Autodesk Inventor part; units mm, degrees
ref_plane "YZ Plane" through (0, 0, 0) normal (1, 0, 0) x (0, 1, 0)
ref_plane "XZ Plane" through (0, 0, 0) normal (0, 1, 0) x (-1, 0, 0)
ref_plane "XY Plane" through (0, 0, 0) normal (0, 0, 1) x (1, 0, 0)
sketch "Sketch1" plane through (0, 0, 0) normal (0, 1, 0) x (-1, 0, 0)
  circle A0 centre (0, 0) radius 22.606
  circle A1 centre (0, 0) radius 25.273
  dimension "d0" = 45.212
  dimension "d1" = 50.546
extrude "Extrusion1" add sketch "Sketch1" along normal mid plane 25.4
sketch "Sketch5" plane through (0, 0, 0) normal (1, 0, 0) x (0, 1, 0)
  line L0 (-12.7, -22.606) -> (12.7, -22.606)
  arc A0 (0, -25.527) -> (0, -19.685) centre (0, -22.606) ccw
  line L1 (0, -25.527) -> (0, -19.685)
  line L2 (0, -25.527) -> (0, -19.685) construction
  point P0 (0, 0)
  dimension "d7" = 2.921
revolve "Revolution2" add sketch "Sketch5" angle 360 about axis through (0, 0, -25.527) along (0, 0, 1)
properties part number "ExternalMotorizedOuterRing" material "PET Plastic"
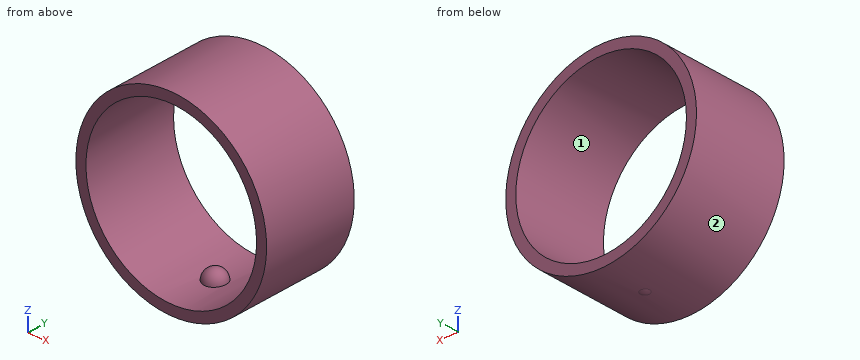
CAD build for the part. Positions are in the model's coordinates, mm. Face numbers are marked on the shaded views. Coordinates: 2 decimals unless noted, no trailing zeros. Order: outer loops, then holes, each group sorted by start corner. A loop starts at its lowest first (then second) coordinate and runs counter-clockwise, first axis right, second up. Notation, with made-up numbers: (-11.75, -26.75) - (15.25, -26.75) arc R29 ccw to (15.25, 6.25) - close; hole circle Ø6 at (85.5, 41.5). An arc over 180 degrees is marked (long way). Use a Markdown table: item, result. Add a question column.
(1) Flat gauge pins, fed straight in: pin 1 (10 mm diameter, centred on x = 19.5, z = 3.5, fed in from +Y); pin 2 (3 mm diameter, centred on x = -17, z = 9, fed in from +Y); pin 3 (1.5 mm diameter, centred on y = -8, z = 11.5, fed in from +X); pin 4 (12 mm diameter, centred on y = 4, z = -8, fed in from -X). Where does each tip first touch, or does it go through?
(2) Drill centre lines: line 1 along Z through (x, y) = (0, 6); line 2 along Z through (x, y) = (12.5, 5.5); line 3 along X through (y, z) = (-6, -5). Where is each one in solid material? Low to high. Write a range as [from, to].
(3) Saw through at A-A (x = 0). Give the cut face in (y, z), then the cut area to 3 significant figures.
(4) Saw through at C-C (z = -12.5). Give the cut face in (x, y), then the cut area to 3 significant figures.
(5) Pull direction Z, two halves, no side cores. Call the marked faces 1 and 2: +Z half, -Z half, draft (parallel to the pull), parting line (faces both ways), or undercut.
(6) Saw through at B-B (z = 0). Give the cut face in (x, y).
(7) Saw through at D-D (y = -7.75). Give the cut face in (x, z).
Solved:
| question | item | result |
|---|---|---|
| 1 | pin 1 | stops at y = 12.7 |
| 1 | pin 2 | passes through |
| 1 | pin 3 | stops at x = 22.87 |
| 1 | pin 4 | stops at x = -25.19 |
| 2 | line 1 | z = [-25.27, -22.61], [22.61, 25.27] |
| 2 | line 2 | z = [-21.97, -18.84], [18.84, 21.97] |
| 2 | line 3 | x = [-24.77, -22.05], [22.05, 24.77] |
| 3 | outline | (-12.7, -25.27) - (-1.19, -25.27) arc R2.92 ccw to (1.19, -25.27) - (12.7, -25.27) - (12.7, -22.61) - (2.92, -22.61) arc R2.92 ccw to (-2.92, -22.61) - (-12.7, -22.61) - close; (-12.7, 22.61) - (12.7, 22.61) - (12.7, 25.27) - (-12.7, 25.27) - close |
| 3 | area | 149 mm² |
| 4 | outline | (-21.97, -12.7) - (-18.84, -12.7) - (-18.84, 12.7) - (-21.97, 12.7) - close; (18.84, -12.7) - (21.97, -12.7) - (21.97, 12.7) - (18.84, 12.7) - close |
| 4 | area | 159 mm² |
| 5 | face 1 | undercut |
| 5 | face 2 | parting line |
| 6 | outline | (-25.27, -12.7) - (-22.61, -12.7) - (-22.61, 12.7) - (-25.27, 12.7) - close; (22.61, -12.7) - (25.27, -12.7) - (25.27, 12.7) - (22.61, 12.7) - close |
| 7 | outline | circle Ø50.55 at (0, 0); hole circle Ø45.21 at (0, 0) |
